Here's how the part is built. I have some questions about the finished solid (model axes, mm). Face numbers are marked on the shaded views. A direction names the side the tool comes from. Round coordinates to 2 decimals unless told otherwise and drop trailing zeros. Order: outer loops, then holes, each group sorted by start corner. A loop starts at its lowest first (then second) coordinate and runs counter-clockwise, first axis right, second up. Notation, with made-up numbers: M 63,36.5 L 88,36.5 A36 cw 88,70.5 Z; hole C 77,81.5 d3. An arc over 180 degrees is marked long. Write item = value, one per line. Start each with the question number.
Item 1: I want a section at C-C, the plane x = -4.5. List the corners of the cut face in (y, z) for me.
Item 2: I want a section at B-B, the plane y = -465. List the corners of the cut face in (x, z) for me, plus the area to 3 significant figures.
Item 3: Please list where these lines run through material, in increasing order: L1, parallel to Y at x = -388, z = 16.5; L2, parallel to Y at x = -254.5, z = -26.5; L3, parallel to X at y = -277.5, z = 27.
Item 4: I want a section at D-D, the plane y = -388.5. List the corners of the cut face in (x, z) for me.
Item 5: We'd pull the mould along Y, two halves only. Please class the marked faces 6, 7 and 8: pulls with the +Y half, pulls with the -Y half, needs draft (parallel to the pull), parting line crosses it, or undercut.
Item 6: I'm going to push flat-ended pins straight in: P1, Ø3, axis at x = -7.5, y = -368.5, coming from the -Z side; P2, Ø10, axis at x = 18.5, z = 16, coming from the -Y side; P3, Ø2, axis at y = -403.5, z = -28.5, coming from the -X side. Where does each tip first touch, or does it pass through?
Item 7: For the marked faces 1, 2, 3, 4 and 5, which set-ups out of +Z, -Z, +X, -X, +Y, -Y let a thin tool reach every point of the face, with its end or its side?
Item 8: I want a section at A-A, the plane z = 0. List the corners of the cut face in (x, y) for me, plus the area to 3 significant figures.
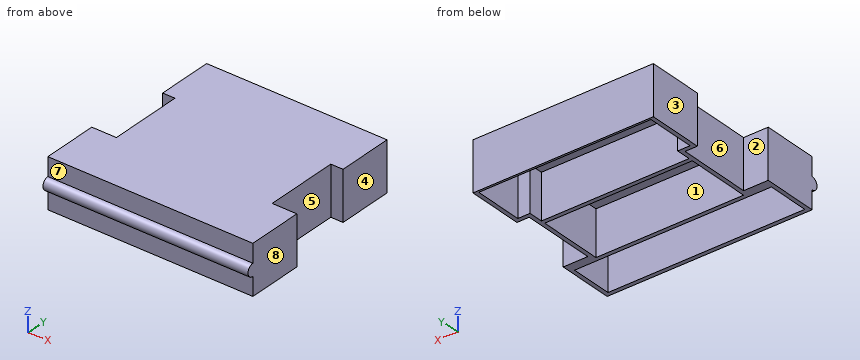
Autodesk Inventor part; units mm, degrees
ref_plane "YZ Plane" through (0, 0, 0) normal (1, 0, 0) x (0, 1, 0)
ref_plane "XZ Plane" through (0, 0, 0) normal (0, 1, 0) x (-1, 0, 0)
ref_plane "XY Plane" through (0, 0, 0) normal (0, 0, 1) x (1, 0, 0)
ref_plane "РабПлоскость1" through (519.783, -178.5074, 484.3845) normal (-0.0032, 1, 0.0035) x (-0.0024, 0.0035, -1)
sketch "Эскиз1" plane through (0, 0, 0) normal (0, 0, 1) x (-1, 0, 0)
  line L0 (0, 0) -> (0, 90)
  line L1 (0, 90) -> (-25, 90)
  line L2 (-25, 90) -> (-75, 90)
  line L3 (-75, 90) -> (-75, 540)
  line L4 (-75, 540) -> (425, 540)
  line L5 (425, 540) -> (425, 90)
  line L6 (425, 90) -> (-75, 90)
  line L7 (175, 315) -> (425, 315)
  line L8 (175, 315) -> (-75, 315)
  line L9 (425, 315) -> (425, 405)
  line L10 (425, 405) -> (365, 405)
  line L11 (365, 405) -> (365, 225)
  line L12 (365, 225) -> (425, 225)
  line L13 (-75, 315) -> (-75, 405)
  line L14 (-75, 405) -> (-15, 405)
  line L15 (-15, 405) -> (-15, 225)
  line L16 (-15, 225) -> (-75, 225)
  line L17 (0, 90) -> (0, 100)
  line L18 (0, 100) -> (-65, 100)
  line L19 (0, 100) -> (415, 100)
  line L20 (425, 540) -> (415, 540)
  line L21 (415, 530) -> (415, 100)
  line L22 (425, 540) -> (425, 530)
  line L23 (415, 530) -> (-65, 530)
  line L24 (-75, 540) -> (-65, 540)
  line L25 (-65, 530) -> (-65, 100)
  point P0 (415, 405)
  point P1 (-65, 405)
  point P2 (-65, 225)
  point P3 (415, 225)
  dimension "d0" = 90
  dimension "d1" = 25
  dimension "d2" = 50
  dimension "d3" = 450
  dimension "d4" = 500
  dimension "d5" = 90
  dimension "d6" = 60
  dimension "d7" = 180
  dimension "d8" = 60
  dimension "d35" = 10
  dimension "d36" = 10
  dimension "d37" = 10
ref_plane "РабПлоскость2" through (0, 0, 60) normal (0, 0, 1) x (1, 0, 0)
extrude "Выдавливание6" add sketch "Эскиз1" along normal mid plane 120 contours L17 L19 L21 L12 L5 L6 | L1 L2 L3 L16 L25 L18 L17 | L10 L21 L23 L25 L14 L3 L4 L5
sketch "Эскиз7" plane through (0, 0, 60) normal (0, 0, 1) x (1, 0, 0)
  line L0 (-415, -100) -> (65, -100)
  line L1 (-415, -100) -> (65, -100)
  line L2 (65, -225) -> (75, -225)
  line L3 (65, -100) -> (65, -225)
  line L4 (65, -225) -> (15, -225)
  line L5 (15, -225) -> (15, -405)
  line L6 (15, -405) -> (65, -405)
  line L7 (-415, -530) -> (65, -530)
  line L8 (65, -405) -> (65, -530)
  line L9 (65, -530) -> (-415, -530)
  line L10 (-415, -530) -> (-415, -405)
  line L11 (-415, -225) -> (-415, -100)
  line L12 (-415, -405) -> (-365, -405)
  line L13 (-365, -405) -> (-365, -225)
  line L14 (-365, -225) -> (-415, -225)
  point P0 (0, 0)
  dimension "d40" = 50
  dimension "d41" = 180
  dimension "d43" = 50
extrude "Выдавливание7" add sketch "Эскиз7" against normal blind 10
sketch "Эскиз8" plane through (0, 0, 50) normal (0, 0, -1) x (-1, 0, 0)
  line L0 (415, -405) -> (415, -530)
  line L1 (365, -225) -> (365, -405)
  line L2 (415, -405) -> (365, -405)
  line L3 (365, -405) -> (365, -225)
  line L4 (415, -100) -> (415, -225)
  line L5 (365, -225) -> (415, -225)
  line L6 (415, -225) -> (415, -220)
  line L7 (415, -220) -> (355, -220)
  line L8 (355, -220) -> (355, -410)
  line L9 (355, -410) -> (415, -410)
  line L10 (415, -410) -> (415, -405)
  line L11 (425, -405) -> (425, -540)
  line L12 (-65, -225) -> (-65, -100)
  line L13 (-65, -225) -> (-15, -225)
  line L14 (-65, -225) -> (-15, -225)
  line L15 (-15, -225) -> (-15, -405)
  line L16 (-15, -405) -> (-65, -405)
  line L17 (-65, -405) -> (-65, -410)
  line L18 (-65, -410) -> (-5, -410)
  line L19 (-5, -410) -> (-5, -220)
  line L20 (-5, -220) -> (-65, -220)
  point P0 (0, 0)
  dimension "d46" = 5
  dimension "d47" = 60
  dimension "d48" = 190
  dimension "d49" = 5
  dimension "d50" = 60
  dimension "d51" = 190
extrude "Выдавливание8" add sketch "Эскиз8" along normal blind 110
sketch "Эскиз9" plane through (0, 0, 50) normal (0, 0, -1) x (-1, 0, 0)
  line L0 (415, -100) -> (415, -220)
  line L1 (415, -100) -> (415, -95)
  line L2 (415, -95) -> (-65, -95)
  line L3 (-65, -220) -> (-65, -100)
  line L4 (-65, -95) -> (-65, -100)
  line L5 (-65, -100) -> (415, -100)
  point P0 (0, 0)
  dimension "d54" = 5
extrude "Выдавливание9" cut sketch "Эскиз9" along normal blind 110
sketch "Эскиз10" plane through (0, 0, 50) normal (0, 0, -1) x (-1, 0, 0)
  line L0 (415, -410) -> (415, -427.5)
  line L1 (415, -410) -> (415, -530)
  line L2 (415, -427.5) -> (-65, -427.5)
  line L3 (-65, -530) -> (-65, -410)
  line L4 (-65, -427.5) -> (-65, -410)
  line L5 (-5, -410) -> (-5, -220)
  line L6 (-65, -410) -> (-5, -410)
  line L7 (-5, -410) -> (-5, -417.5)
  line L8 (-5, -417.5) -> (355, -417.5)
  line L9 (355, -410) -> (415, -410)
  line L10 (355, -417.5) -> (355, -410)
  line L11 (355, -410) -> (415, -410)
  point P0 (0, 0)
  dimension "d57" = 17.5
  dimension "d58" = 480
  dimension "d59" = 7.5
extrude "Выдавливание10" add sketch "Эскиз10" along normal blind 110
sketch "Эскиз11" plane through (0, 0, 50) normal (0, 0, -1) x (-1, 0, 0)
  line L0 (355, -220) -> (355, -417.5)
  line L1 (355, -220) -> (355, -260)
  line L2 (355, -260) -> (-5, -260)
  line L3 (-5, -220) -> (-5, -417.5)
  line L4 (-5, -260) -> (-5, -250)
  line L5 (-5, -250) -> (355, -250)
  point P0 (0, 0)
  dimension "d62" = 40
  dimension "d63" = 10
extrude "Выдавливание11" add sketch "Эскиз11" along normal blind 110
sketch "Эскиз12" plane through (0, 0, 60) normal (0, 0, 1) x (1, 0, 0)
  line L0 (15, -225) -> (75, -225)
  line L1 (75, -90) -> (-425, -90)
  line L2 (75, -225) -> (45, -225)
  line L3 (45, -225) -> (45, -90)
  line L4 (45, -90) -> (75, -90)
  line L5 (75, -90) -> (75, -225)
  line L6 (-425, -225) -> (-365, -225)
  line L7 (-425, -225) -> (-395, -225)
  line L8 (-395, -225) -> (-395, -90)
  line L9 (-395, -90) -> (-425, -90)
  line L10 (-425, -90) -> (-425, -225)
  point P0 (0, 0)
  dimension "d66" = 30
extrude "Выдавливание12" cut sketch "Эскиз12" against normal blind 120
sketch "Эскиз13" plane through (0, 0, 50) normal (0, 0, -1) x (-1, 0, 0)
  line L0 (-45, -95) -> (-45, -220)
  line L1 (395, -95) -> (-45, -95)
  line L2 (-45, -220) -> (-35, -220)
  line L3 (-35, -220) -> (-35, -95)
  line L4 (-35, -95) -> (-45, -95)
  line L5 (-45, -95) -> (-45, -220)
  line L6 (395, -95) -> (385, -95)
  line L7 (385, -95) -> (385, -220)
  line L8 (385, -220) -> (395, -220)
  line L9 (395, -220) -> (395, -95)
  point P0 (0, 0)
  dimension "d69" = 10
  dimension "d70" = 10
extrude "Выдавливание13" add sketch "Эскиз13" along normal blind 110
sketch "Эскиз14" plane through (0, 0, -60) normal (0, 0, -1) x (-1, 0, 0)
  point P0 (0, 0)
sketch "Эскиз15" plane through (75, -540, 60) normal (1, 0, 0) x (0, 0, -1)
  line L0 (0, 135) -> (0, 0)
  line L1 (120, 0) -> (120, 135)
  line L2 (0, 0) -> (120, 0)
  line L3 (120, 0) -> (60, 0)
  arc A0 (45, 0) -> (75, 0) centre (60, 0) ccw
  point P0 (60, 540)
  dimension "d73" = 60
  dimension "d74" = 30
extrude "Выдавливание14" add sketch "Эскиз15" against normal blind 500
sketch "Эскиз16" plane through (0, 0, 50) normal (0, 0, -1) x (-1, 0, 0)
  line L0 (-35, -220) -> (-35, -95)
  line L1 (-35, -220) -> (-35, -215)
  line L2 (-35, -215) -> (-5, -215)
  line L3 (-5, -220) -> (-35, -220)
  line L4 (-5, -215) -> (-5, -220)
  line L5 (-5, -220) -> (-35, -220)
  line L6 (385, -220) -> (355, -220)
  line L7 (355, -220) -> (355, -215)
  line L8 (355, -215) -> (385, -215)
  line L9 (385, -95) -> (385, -220)
  line L10 (385, -215) -> (385, -220)
  line L11 (355, -220) -> (385, -220)
  point P0 (0, 0)
  dimension "d77" = 5
extrude "Выдавливание15" add sketch "Эскиз16" along normal blind 110
properties part number "ОсноваКорпуса" material "Титан"
Filled in:
q1.outline = M -540,-60 L -530,-60 L -530,50 L -427.5,50 L -427.5,-60 L -417.5,-60 L -417.5,50 L -260,50 L -260,-60 L -250,-60 L -250,50 L -95,50 L -95,-60 L -90,-60 L -90,60 L -540,60 L -540,15 A15 ccw -540,-15 Z
q2.outline = M -425,-60 L -415,-60 L -415,50 L 65,50 L 65,-60 L 75,-60 L 75,60 L -425,60 Z
q2.area = 7,200 mm^2
q3.L1 = -540 to -530, -427.5 to -405, -225 to -90
q3.L2 = -540 to -530, -427.5 to -417.5, -260 to -250, -95 to -90
q3.L3 = -365 to -355, 5 to 15
q4.outline = M -365,-60 L -355,-60 L -355,50 L 5,50 L 5,-60 L 15,-60 L 15,60 L -365,60 Z
q5.face_6 = undercut
q5.face_7 = pulls with the -Y half
q5.face_8 = needs draft
q6.P1 = 50
q6.P2 = -550.2
q6.P3 = -365
q7.face_1 = -Z
q7.face_2 = +Z, -Z, -X
q7.face_3 = +Z, -Z, -X, +Y
q7.face_4 = +Z, -Z, +X, +Y
q7.face_5 = +Z, -Z, +X
q8.outline = M -425,-555 L 75,-555 L 75,-405 L 15,-405 L 15,-225 L 45,-225 L 45,-90 L -395,-90 L -395,-225 L -365,-225 L -365,-405 L -425,-405 Z; hole M -415,-530 L 65,-530 L 65,-427.5 L -415,-427.5 Z; hole M -385,-215 L -355,-215 L -355,-250 L 5,-250 L 5,-215 L 35,-215 L 35,-95 L -385,-95 Z; hole M -355,-417.5 L 5,-417.5 L 5,-260 L -355,-260 Z
q8.area = 33,900 mm^2
